The model under review builds one solid part; all positions refer to its coordinate system, in mm. A direction names the side the tool comes from. Coordinates: 2 decimals unless noted, no trailing zeros. Order: outer loops, then holes, each group sorted by start corner. A loop starts at its lowest first (then second) coordinate and runs counter-clockwise, first axis right, second up. Notation, with made-up numbers: (-11, 52) -> (17, 52) arc R18 ccw to (17, 85) -> close; hole circle Ø3 at (-14.5, 26). An arc over 180 degrees is marked (long way). Put each result on its own line as item: value.
Autodesk Inventor part; units mm, degrees
ref_plane "YZ Plane" through (0, 0, 0) normal (1, 0, 0) x (0, 1, 0)
ref_plane "XZ Plane" through (0, 0, 0) normal (0, 1, 0) x (-1, 0, 0)
ref_plane "XY Plane" through (0, 0, 0) normal (0, 0, 1) x (1, 0, 0)
sketch "スケッチ1" plane through (0, 0, 0) normal (0, 0, 1) x (1, 0, 0)
  line L0 (12.5, -5.5) -> (-12.5, -5.5)
  line L1 (-12.5, -5.5) -> (-12.5, 5.5)
  line L2 (-12.5, 5.5) -> (12.5, 5.5)
  line L3 (12.5, 5.5) -> (12.5, -5.5)
  line L4 (12.5, -5.5) -> (-12.5, 5.5) construction
  line L5 (-12.5, -5.5) -> (12.5, 5.5) construction
  circle A0 centre (10, -2.5) radius 1.85
  circle A1 centre (-10, -2.5) radius 1.85
  line L6 (12.5, -4.5) -> (-12.5, -4.5)
  line L7 (12.5, 4.5) -> (-12.5, 4.5)
  line L8 (4, -4.5) -> (4, 4.5)
  line L9 (-4, -4.5) -> (-4, 4.5)
  line L10 (4.8, -4.5) -> (4.8, 4.5)
  line L11 (-4.8, -4.5) -> (-4.8, 4.5)
  line L12 (7.5, -4.5) -> (7.5, 4.5)
  line L13 (6.7, -4.5) -> (6.7, 4.5)
  line L14 (-7.5, -4.5) -> (-7.5, 4.5)
  line L15 (-6.7, -4.5) -> (-6.7, 4.5)
  point P0 (0, 0)
  dimension "d0" = 25
  dimension "d1" = 11
  dimension "d2" = 3.7
  dimension "d3" = 3.7
extrude "押し出し1" add sketch "スケッチ1" along normal blind 8.1 contours L0 L1 L6 L3 | L6 L12 L7 L3 | L1 L7 L14 L6 | L7 L1 L2 L3 | L6 L8 L7 L10 | L11 L7 L9 L6
properties part number "griper_base_TPU-2" material "ゴム、シリコーン"
Item 1: Consider section A-A on y = 1.75. Write out the cut boundary in (x, z), and give its area (3 significant figures).
Answers below:
outline: (-12.5, 0) -> (-7.5, 0) -> (-7.5, 8.1) -> (-12.5, 8.1) -> close; (-4.8, 0) -> (-4, 0) -> (-4, 8.1) -> (-4.8, 8.1) -> close; (4, 0) -> (4.8, 0) -> (4.8, 8.1) -> (4, 8.1) -> close; (7.5, 0) -> (12.5, 0) -> (12.5, 8.1) -> (7.5, 8.1) -> close
area: 94.0 mm^2
Item 2: For line 1 (X direction, y = 1, z = 5); line 2 (Y direction, x = 1.75, z = 5.5); line 3 (Y direction, x = -10, z = 6), list the stretches that pass through material, from the lowest coordinate up. Write a range as from..to.
Answers below:
line 1: -12.5..-7.5, -4.8..-4, 4..4.8, 7.5..12.5
line 2: -5.5..-4.5, 4.5..5.5
line 3: -5.5..-4.35, -0.65..5.5
Item 3: For faces 1 (the flat face through (-12.5, 0, 4)), 2 (the flat face through (4, 0, 4)), list the 3-axis set-ups (+Z, -Z, +X, -X, +Y, -Y) from which the entire face can be reached by the end or side of a thin tool; tool diameter is ignored.
Answers below:
face 1: +Z, -Z, -X, +Y, -Y
face 2: +Z, -Z
Item 4: Consider section D-D on y = -2.5. Write out the cut boundary in (x, z), and give its area (3 significant figures).
Answers below:
outline: (-12.5, 0) -> (-11.85, 0) -> (-11.85, 8.1) -> (-12.5, 8.1) -> close; (-8.15, 0) -> (-7.5, 0) -> (-7.5, 8.1) -> (-8.15, 8.1) -> close; (-4.8, 0) -> (-4, 0) -> (-4, 8.1) -> (-4.8, 8.1) -> close; (4, 0) -> (4.8, 0) -> (4.8, 8.1) -> (4, 8.1) -> close; (7.5, 0) -> (8.15, 0) -> (8.15, 8.1) -> (7.5, 8.1) -> close; (11.85, 0) -> (12.5, 0) -> (12.5, 8.1) -> (11.85, 8.1) -> close
area: 34.0 mm^2
Item 5: Consider section C-C on z = 3. Write out the cut boundary in (x, y).
Answers below:
outline: (-12.5, -5.5) -> (12.5, -5.5) -> (12.5, 5.5) -> (-12.5, 5.5) -> close; hole circle Ø3.7 at (-10, -2.5); hole (-7.5, -4.5) -> (-4.8, -4.5) -> (-4.8, 4.5) -> (-7.5, 4.5) -> close; hole (-4, -4.5) -> (4, -4.5) -> (4, 4.5) -> (-4, 4.5) -> close; hole (4.8, -4.5) -> (7.5, -4.5) -> (7.5, 4.5) -> (4.8, 4.5) -> close; hole circle Ø3.7 at (10, -2.5)
Item 6: Consider section B-B on x = 0. Write out the cut boundary in (y, z), and give its area (3 significant figures).
Answers below:
outline: (-5.5, 0) -> (-4.5, 0) -> (-4.5, 8.1) -> (-5.5, 8.1) -> close; (4.5, 0) -> (5.5, 0) -> (5.5, 8.1) -> (4.5, 8.1) -> close
area: 16.2 mm^2
Item 7: Mouldability with a two-part tool opening along Y and no side actions: class faces 3 (the flat face through (6, 4.5, 4)), 4 (the flat face through (12.5, 0, 4)), 5 (the flat face through (0, -5.5, 4)) as +Y half, -Y half, draft (parallel to the pull), parting line (faces both ways), or undercut.
Answers below:
face 3: undercut
face 4: draft
face 5: -Y half
